Work out the finished part from the listing and answer in its coordinate system (mm). A direction names the side the tool comes from. Round coordinates to 2 decimals unless told otherwise and drop trailing zeros. Return JSON: item names as keys, results as strings.
from build123d import *

# Parameters (mm, degrees)
SKETCH1_W           = 100
SKETCH1_H           = 100
BOSS_EXTRUDE1_DEPTH = 4
SKETCH3_R           = 2
CUT_EXTRUDE1_DEPTH  = 2
CUT_EXTRUDE2_DEPTH  = 2


with BuildPart() as part:
    # Sketch1 → Boss-Extrude1 (new body)
    with BuildSketch(Plane(origin=(0, 0, 0), x_dir=(1, 0, 0), z_dir=(0, 1, 0))):
        with Locations((15.12345679, -26.466049383)):
            Rectangle(SKETCH1_W, SKETCH1_H)
    extrude(amount=BOSS_EXTRUDE1_DEPTH)

    # Sketch3 → Cut-Extrude1 (cut)
    with BuildSketch(Plane(origin=(0, 4, 0), x_dir=(1, 0, 0), z_dir=(0, 1, 0))):
        with Locations((-4.87654321, -26.466049383)):
            Circle(SKETCH3_R)
        with Locations((10.12345679, -26.466049383)):
            Circle(SKETCH3_R)
    extrude(amount=-CUT_EXTRUDE1_DEPTH, mode=Mode.SUBTRACT)

    # Sketch5 → Cut-Extrude2 (cut)
    with BuildSketch(Plane.XZ):
        Polygon((-0.835091326, 26.466049383), (-2.855817268, 29.966049383), (-6.897269152, 29.966049383), (-8.917995094, 26.466049383), (-6.897269152, 22.966049383), (-2.855817268, 22.966049383), align=None)
        Polygon((14.164908674, 26.466049383), (12.144182732, 29.966049383), (8.102730848, 29.966049383), (6.082004906, 26.466049383), (8.102730848, 22.966049383), (12.144182732, 22.966049383), align=None)
    extrude(amount=-CUT_EXTRUDE2_DEPTH, mode=Mode.SUBTRACT)


solid = part.part
1) A flat-ended cylindrical pin translates along its axis: pin 1 (5 mm diameter, centred on x = -4.88, z = 26.47, fed in from -Y). Find the tip coordinate at first contact, or state that the pin passes through.
Verdict:
{"pin 1": "stops at y = 2"}
2) Determine the mould class of faces 1 (the cylindrical face through (-5.137, 3.014, 24.483)), 2 (the flat face through (14, 2, 76.466)), 3 (the flat face through (14.4, 0, 25.8)), 4 (the flat face through (12, 2, 28)) for opening direction Z: pulls with the +Z half, pulls with the -Z half, needs draft (parallel to the pull), parting line crosses it, or undercut.
Verdict:
{"face 1": "undercut", "face 2": "pulls with the +Z half", "face 3": "needs draft", "face 4": "undercut"}
3) Find the intervals of material crossed by L1, parallel to Z at x = 10.5, y = 3.5, in increasing order.
Verdict:
{"L1": "z = -23.53 to 24.5, 28.43 to 76.47"}
4) A tool of negligible diameter and unlimited length cuts with its end or side. For faces 5 (the flat face through (-3, 2, 28)), 6 (the flat face through (-34.877, 2, 27)), from which of +Z, -Z, +X, -X, +Y, -Y can it reach the whole face along a straight path? Write none if from no direction.
Verdict:
{"face 5": "-Y", "face 6": "+Z, -Z, -X, +Y, -Y"}
